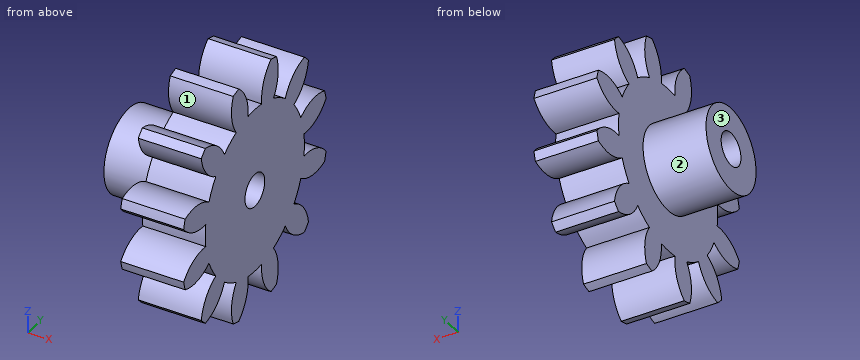
from build123d import *

# Parameters (mm, degrees)
BASPROSKE_W         = 3.81
BASPROSKE_H         = 7.408333333
TOOTHCUT_DEPTH      = 12.148224323
TEETHCUTS_COUNT     = 12
TEETHCUTS_ANGLE     = 330
BORSKE_R            = 5.0038
BORE_DEPTH          = 50.8000508
SKETCH1_R           = 5.0038
BOSS_EXTRUDE1_DEPTH = 3.81
SKETCH2_R           = 2.54
BOSS_EXTRUDE2_DEPTH = 3.81
SKETCH3_R           = 1.0033
CUT_EXTRUDE1_DEPTH  = 13.746829501


with BuildPart() as part:
    # BasProSke → Base-Revolve (revolve)
    with BuildSketch(Plane(origin=(0, 0, 0), x_dir=(1, 0, 0), z_dir=(0, 1, 0)), mode=Mode.PRIVATE) as base_revolve_sk:
        with Locations((1.905, 3.704166667)):
            Rectangle(BASPROSKE_W, BASPROSKE_H)
    revolve(base_revolve_sk.sketch.rotate(Axis((-10, 0, 0), (1, 0, 0)), 180), axis=Axis((-10, 0, 0), (1, 0, 0)))

    # TooCutSke → ToothCut (cut, through all)
    with BuildSketch(Plane(origin=(0, 0, 0), x_dir=(0, 0, -1), z_dir=(1, 0, 0))):
        with BuildLine():
            ThreePointArc((0.69063345, 4.981553782), (0, 5.0292), (-0.69063345, 4.981553782))
            ThreePointArc((-0.69063345, 4.981553782), (-0.883041418, 6.239186652), (-1.661175181, 7.245749671))
            ThreePointArc((-1.661175181, 7.245749671), (0, 7.433733333), (1.661175181, 7.245749671))
            ThreePointArc((1.661175181, 7.245749671), (0.883041418, 6.239186652), (0.69063345, 4.981553782))
        make_face()
    toothcut = extrude(amount=TOOTHCUT_DEPTH, mode=Mode.SUBTRACT)

    # TeethCuts: ToothCut ×12 about axis
    teethcuts_axis = Axis((-10, 0, 0), (1, 0, 0))
    for i in range(1, TEETHCUTS_COUNT):
        add(toothcut.rotate(teethcuts_axis, i * TEETHCUTS_ANGLE / (TEETHCUTS_COUNT - 1)), mode=Mode.SUBTRACT)

    # BorSke → Bore (cut, symmetric)
    with BuildSketch(Plane(origin=(0, 0, 0), x_dir=(0, 0, -1), z_dir=(1, 0, 0))):
        with Locations(Location((0, 0, 0), (0, 0, 180))):
            Circle(BORSKE_R)
    extrude(amount=BORE_DEPTH, both=True, mode=Mode.SUBTRACT)

    # Sketch1 → Boss-Extrude1 (add)
    with BuildSketch(Plane(origin=(0, 0, 0), x_dir=(0, 0, -1), z_dir=(1, 0, 0))):
        Circle(SKETCH1_R)
    extrude(amount=BOSS_EXTRUDE1_DEPTH)

    # Sketch2 → Boss-Extrude2 (add)
    with BuildSketch(Plane.ZY):
        with Locations(Location((0, 0, 0), (0, 0, 180))):
            Circle(SKETCH2_R)
    extrude(amount=BOSS_EXTRUDE2_DEPTH)

    # Sketch3 → Cut-Extrude1 (cut, through all)
    with BuildSketch(Plane.ZY.offset(3.81)):
        Circle(SKETCH3_R)
    extrude(amount=-CUT_EXTRUDE1_DEPTH, mode=Mode.SUBTRACT)


solid = part.part
Check sheet for the modelled part. Datum: model origin and axes. Units: mm. Face numbers are marked on the shaded views. Round coordinates to 2 decimals unless told otherwise and drop trailing zeros. Order: outer loops, then holes, each group sorted by start corner. A loop starts at its lowest first (then second) coordinate and runs counter-clockwise, first axis right, second up.
Q1. Cross-section at C-C, the plane x = -2.5. Enter the section's corners in (y, z), plus the area to 3 significant figures.
Filled sheet:
outline: circle Ø5.08 at (0, 0); hole circle Ø2.01 at (0, 0)
area: 17.1 mm2
Q2. Cross-section at A-A, the plane z = 0. Enter the section's corners in (x, y), plus the area to 3 significant figures.
Filled sheet:
outline: (-3.81, -2.54) - (0, -2.54) - (0, -5.03) - (3.81, -5.03) - (3.81, -1) - (-3.81, -1) - close; (-3.81, 1) - (3.81, 1) - (3.81, 5.03) - (0, 5.03) - (0, 2.54) - (-3.81, 2.54) - close
area: 42.4 mm2
Q3. Depth check by flat-ended pin: P1, Ø1, axis at x = -2.5, z = 3.5, coming from the +Y side; P2, Ø5, axis at y = 2.5, z = 4.5, coming from the +X side; P3, Ø3, axis at x = 3, y = 0, coming from the -Z side. Enter the tip coordinate at first touch or a pass-through.
Filled sheet:
P1: passes through
P2: stops at x = 3.81
P3: stops at z = -7.11
Q4. Draft check along Z on the marked faces 1, 2 and 3. Enter one of: pulls with the +Z half, pulls with the -Z half, needs draft (parallel to the pull), parting line crosses it, or undercut.
Filled sheet:
face 1: undercut
face 2: parting line crosses it
face 3: needs draft
Q5. Cross-section at D-D, the plane z = 5.75. Enter the section's corners in (x, y), plus the area to 3 significant figures.
Filled sheet:
outline: (0, -2.34) - (3.81, -2.34) - (3.81, -0.73) - (0, -0.73) - close; (0, 0.73) - (3.81, 0.73) - (3.81, 2.34) - (0, 2.34) - close
area: 12.3 mm2
Q6. Scan lines: L1, parallel to Y at x = -2.5, z = 0; L2, parallel to Z at x = 1.25, y = -4.25; L3, parallel to X at y = 4, z = 3.25. Record each from-to range of solid material in increasing order.
Filled sheet:
L1: y = -2.54 to -1, 1 to 2.54
L2: z = -5.19 to -3.24, -2.69 to 2.69, 3.24 to 5.19
L3: x = 0 to 3.81
